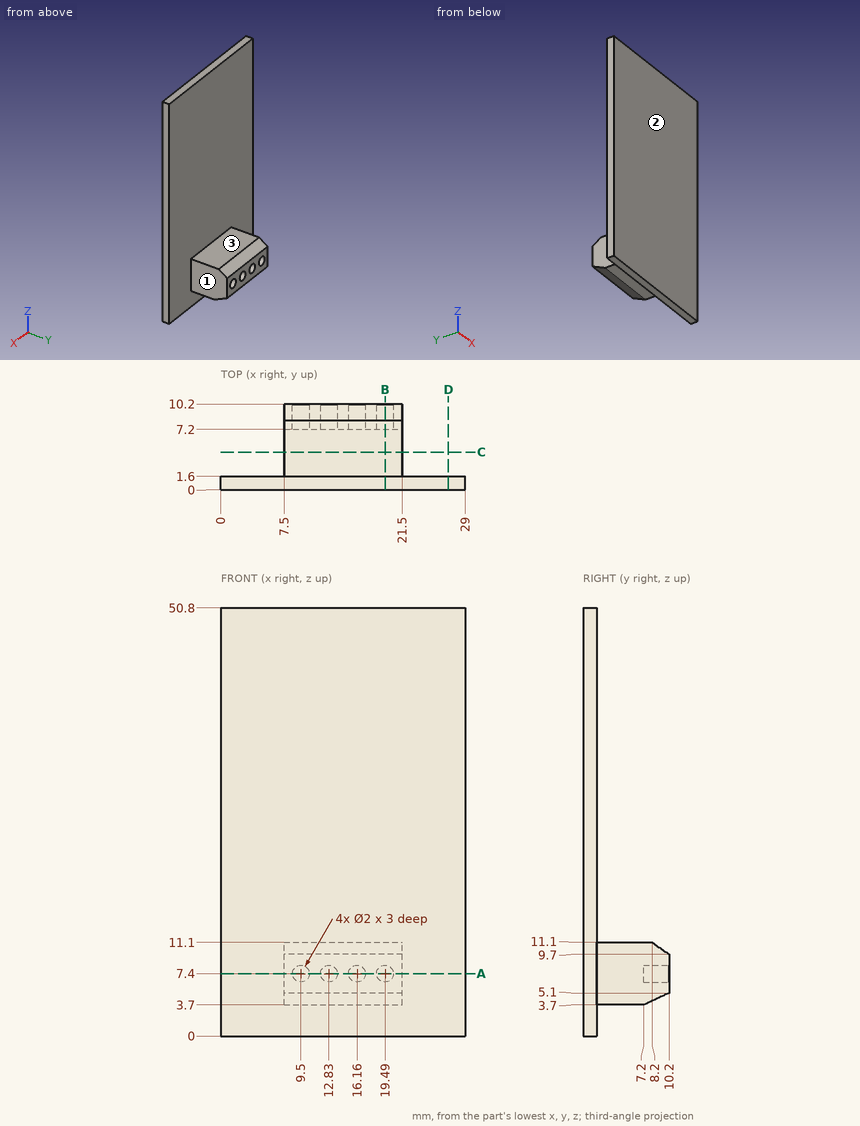
Design review of the part shown in the three views and the two pictorial views. Dimensions are in mm from the part's minimum x, y and z. A direction names the side the tool comes from. Coordinates: 2 decimals unless noted, no trailing zeros. Write each loop counter-clockwise with the first axis right and the second up, starting at its lowest first coordinate (ties: lowest second). Pieces come first, ordered by that corner, then holes.
1) To check wall thickness, follow probe 1 along X at (y, z) = (8.5, 7.4); probe 2 along Y at (x, z) = (21.5, 20); probe 3 along Z at (x, y) = (16.16, 8.5). State the ranges of each line that lie inside material, in increasing order.
2) We need section A-A on z = 7.4. State the section outline as (x, y) points, then the cut area to 3 significant figures.
3) We need section B-B on x = 19.49. State the section outline as (y, z) points.
4) Machinability: for the marked faces 1, 2 and 3, which of the approach directions +Z, -Z, +X, -X, +Y, -Y give a long, thin tool a straight path to every point of the face, cutting with its end or side? Answer none if there is none.
5) We need section D-D on x = 27. State the section outline as (y, z) points.
6) We need section C-C on y = 4.5. State the section outline as (x, z) points.
7) Clearance check with flat-ended pins moving along their axes: pin 1 Ø2 at (x, z) = (13, 7.5) entering from +Y; pin 2 Ø1.6 at (x, z) = (16.16, 7.4) entering from +Y; pin 3 Ø2 at (y, z) = (4, 6.5) entering from +X; pin 4 Ø3.5 at (y, z) = (4, 7.5) entering from -X. State where each tip first meets the part, or that it passes through.
Answer list:
1. probe 1: x = 7.5 to 8.5, 10.5 to 11.83, 13.83 to 15.16, 17.16 to 18.49, 20.49 to 21.5
1. probe 2: y = 0 to 1.6
1. probe 3: z = 4.31 to 6.4, 8.4 to 10.89
2. outline: (0, 0) - (29, 0) - (29, 1.6) - (21.5, 1.6) - (21.5, 10.2) - (20.49, 10.2) - (20.49, 7.2) - (18.49, 7.2) - (18.49, 10.2) - (17.16, 10.2) - (17.16, 7.2) - (15.16, 7.2) - (15.16, 10.2) - (13.83, 10.2) - (13.83, 7.2) - (11.83, 7.2) - (11.83, 10.2) - (10.5, 10.2) - (10.5, 7.2) - (8.5, 7.2) - (8.5, 10.2) - (7.5, 10.2) - (7.5, 1.6) - (0, 1.6) - close
2. area: 143 mm2
3. outline: (0, 0) - (1.6, 0) - (1.6, 3.7) - (7.2, 3.7) - (10.2, 5.1) - (10.2, 6.4) - (7.2, 6.4) - (7.2, 8.4) - (10.2, 8.4) - (10.2, 9.7) - (8.2, 11.1) - (1.6, 11.1) - (1.6, 50.8) - (0, 50.8) - close
4. face 1: +Z, -Z, +X, +Y
4. face 2: +Z, -Z, +X, -X, -Y
4. face 3: +Z, +X, -X, +Y
5. outline: (0, 0) - (1.6, 0) - (1.6, 50.8) - (0, 50.8) - close
6. outline: (7.5, 3.7) - (21.5, 3.7) - (21.5, 11.1) - (7.5, 11.1) - close
7. pin 1: stops at y = 10.2
7. pin 2: stops at y = 7.2
7. pin 3: stops at x = 21.5
7. pin 4: stops at x = 7.5
